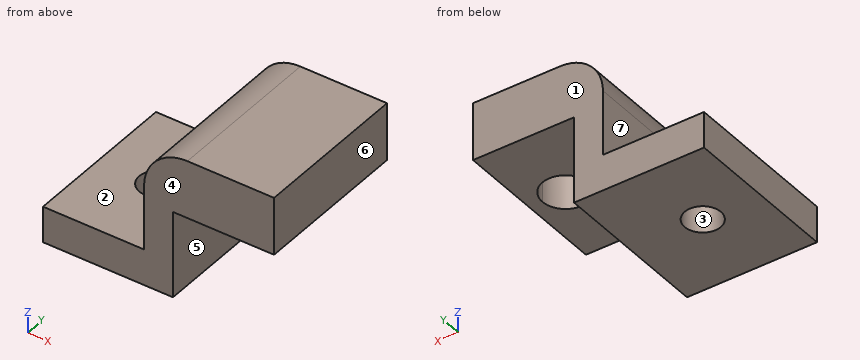
```python
from build123d import *

# Parameters (mm, degrees)
F1_DEPTH = 27.94
F3_DEPTH = 7.62
F4_R     = 7.62
F5_R     = 3.175
F6_DEPTH = 25.4


with BuildPart() as f1:
    # F0 (on Front) → F1 (new body)
    with BuildSketch(Plane.XZ):
        Polygon((-22.86, 0), (0, 0), (0, 15.24), (17.78, 15.24), (17.78, 25.4), (-5.08, 25.4), (-5.08, 6.35), (-22.86, 6.35), align=None)
    extrude(amount=F1_DEPTH)

    # F2 (on face) → F3 (cut)
    with BuildSketch(Plane(origin=(0, 0, 15.24), x_dir=(1, 0, 0), z_dir=(0, 0, -1))):
        with BuildLine():
            ThreePointArc((11.43, 9.906), (14.303682, 11.096318), (15.494, 13.97))
            ThreePointArc((15.494, 13.97), (14.303682, 16.843682), (11.43, 18.034))
            Line((11.43, 18.034), (11.43, 9.906))
        make_face()
        with BuildLine():
            Line((11.43, 9.906), (11.43, 18.034))
            ThreePointArc((11.43, 18.034), (7.366, 13.97), (11.43, 9.906))
        make_face()
    extrude(amount=-F3_DEPTH, mode=Mode.SUBTRACT)

    # F4
    f4_edges = [f1.edges().sort_by_distance(p)[0] for p in [
        (-5.08, -13.97, 25.4),
    ]]
    fillet(f4_edges, radius=F4_R)

    # F5 (on face) → F6 (cut)
    with BuildSketch(Plane(origin=(0, 0, 0), x_dir=(1, 0, 0), z_dir=(0, 0, -1))):
        with Locations((-12.7, 13.97)):
            Circle(F5_R)
    extrude(amount=-F6_DEPTH, mode=Mode.SUBTRACT)


solid = f1.part
```
For this review, take the finished solid that the model builds, in its own axes (mm). Face numbers are marked on the shaded views. A direction names the side the tool comes from. Coordinates: 2 decimals unless noted, no trailing zeros. Write each loop counter-clockwise with the first axis right and the second up, starting at its lowest first coordinate (ties: lowest second). Pieces come first, ordered by that corner, then holes. Notation, with made-up numbers: (8.25, 16.25) - (40.25, 16.25) arc R22 cw to (40.25, 25.25) - close; hole circle Ø10 at (-36.75, 41). An arc over 180 degrees is marked (long way). Answer in a Markdown table with one row per item. Add a question column.
Q1. Draft analysis for pull direction Y (two halves, no side actions). For the marked faces 1, 2, 3 and 4, state which applies: +Y half, -Y half, draft (parallel to the pull), parting line (faces both ways), or undercut.
Q2. For P1, Ø5, axis at x = 11, z = 14, coming from the +Y side; P2, Ø3, axis at x = -9.5, y = -6.5, coming from the +Z side; P3, Ø5, axis at x = -12.7, y = -13.97, coming from the -Z side; P4, Ø9, axis at x = 12.5, y = -18.5, coming from the -Z side, all flat-tipped, find the tip position at first contact; note any pin that passes through.
Q3. We need section A-A, the plane x = -12.7. State the section outline as (y, z) points (3 decimals).
Q4. We need section C-C, the plane z = 3. State the section outline as (x, y) points (3 decimals).
Q5. We need section D-D, the plane z = 11.5. State the section outline as (x, y) points, and give its area (3 significant figures).
Q6. We need section B-B, the plane y = -22. State the section outline as (x, z) points.
Q7. For probe 1 along Y at (x, z) = (-12.7, 2.25) (3 decimals); probe 2 along X at (y, z) = (-13.97, 4.25) (3 decimals); probe 3 along Z at (x, y) = (-6, -1.5), list the stretches that pass through material, from the lowest coordinate up.
Q8. Tool access review of the marked faces 5, 6 and 7: name each direction out of +Z, -Z, +X, -X, +Y, -Y from which nothing blocks a thin tool from reaching the whole face with its end or side.
Answer list:
| question | item | result |
|---|---|---|
| 1 | face 1 | +Y half |
| 1 | face 2 | draft |
| 1 | face 3 | undercut |
| 1 | face 4 | -Y half |
| 2 | P1 | stops at y = 0 |
| 2 | P2 | stops at z = 6.35 |
| 2 | P3 | passes through |
| 2 | P4 | stops at z = 15.24 |
| 3 | outline | (-27.94, 0) - (-17.145, 0) - (-17.145, 6.35) - (-27.94, 6.35) - close; (-10.795, 0) - (0, 0) - (0, 6.35) - (-10.795, 6.35) - close |
| 4 | outline | (-22.86, -27.94) - (0, -27.94) - (0, 0) - (-22.86, 0) - close; hole circle Ø6.35 at (-12.7, -13.97) |
| 5 | outline | (-5.08, -27.94) - (0, -27.94) - (0, 0) - (-5.08, 0) - close |
| 5 | area | 142 mm2 |
| 6 | outline | (-22.86, 0) - (0, 0) - (0, 15.24) - (17.78, 15.24) - (17.78, 25.4) - (2.54, 25.4) arc R7.62 ccw to (-5.08, 17.78) - (-5.08, 6.35) - (-22.86, 6.35) - close |
| 7 | probe 1 | y = -27.94 to -17.145, -10.795 to 0 |
| 7 | probe 2 | x = -22.86 to -15.875, -9.525 to 0 |
| 7 | probe 3 | z = 0 to 6.35 |
| 8 | face 5 | -Z, +X, +Y, -Y |
| 8 | face 6 | +Z, -Z, +X, +Y, -Y |
| 8 | face 7 | +Z, -X, +Y, -Y |
